from build123d import *

# Parameters (mm, degrees)
F0_R     = 2
F1_DEPTH = 3
F2_R     = 4
F3_DEPTH = 2


with BuildPart() as f1:
    # F0 (on Front) → F1 (new body)
    with BuildSketch(Plane.XZ):
        with BuildLine():
            ThreePointArc((0, 5), (1.464466, 1.464466), (5, 0))
            Line((5, 0), (70, 0))
            ThreePointArc((70, 0), (73.535534, 1.464466), (75, 5))
            Line((75, 5), (75, 20))
            ThreePointArc((75, 20), (73.535534, 23.535534), (70, 25))
            Line((70, 25), (5, 25))
            ThreePointArc((5, 25), (1.464466, 23.535534), (0, 20))
            Line((0, 20), (0, 5))
        make_face()
        with Locations((5, 5)):
            Circle(F0_R, mode=Mode.SUBTRACT)
        with Locations((70, 20)):
            Circle(F0_R, mode=Mode.SUBTRACT)
    extrude(amount=F1_DEPTH)

    # F2 (on face) → F3 (cut)
    with BuildSketch(Plane.XZ.offset(3)):
        with Locations((5, 5)):
            Circle(F2_R)
        with Locations((70, 20)):
            Circle(F2_R)
    extrude(amount=-F3_DEPTH, mode=Mode.SUBTRACT)


solid = f1.part
Check sheet for the modelled part. Datum: model origin and axes. Units: mm. A direction names the side the tool comes from. Give positions to 0.01 mm unless a question says otherwise; leave off trailing zeros. Write each loop counter-clockwise with the first axis right and the second up, starting at its lowest first coordinate (ties: lowest second). Pieces come first, ordered by that corner, then holes. Notation, with made-up numbers: (41.25, 7.25) -> (49.25, 7.25) arc R16 cw to (49.25, 13.25) -> close; hole circle Ø11 at (21.25, 5.25). An arc over 180 degrees is marked (long way). Use one line per item in the form item = value. Start each with the question number.
1. Thickness scan on line 1 along Z through (x, y) = (5, -0.4); line 2 along X through (y, z) = (-0.35, 20); line 3 along Z through (x, y) = (5, -1.95). Record the ranges inside material, lowest first. Write a range as from..to.
2. Mould release check, pull along Z, two halves, no side actions. Record for faces 3 (the flat face through (6, -1, 7)), 4 (the flat face through (37, 0, 13)), 5 (the flat face through (68, -1, 19)), 6 (the cylindrical face through (74, -1, 23)): pulls with the +Z half, pulls with the -Z half, needs draft (parallel to the pull), parting line crosses it, or undercut.
3. Section check A-A (y = -0.5). Record the cut outline in (x, z).
4. Access from +Z, -Z, +X, -X, +Y, -Y to the whole of each face (thin tool, end or side, straight path). Record for faces 1 (the flat face through (0, -1, 13)), 2 (the cylindrical face through (73.815, -2.014, 21.201)).
5. Section check B-B (z = 21). Record the cut outline in (x, y).
6. Go/stop test with flat-tipped pins: P1, Ø4, axis at x = 70, z = 21.5, coming from the -Y side; P2, Ø3, axis at x = 5, z = 5, coming from the +Y side (3 decimals). Record where each tip stops, or that it passes through.
Conclusion:
q1.line_1 = 0..3, 7..25
q1.line_2 = 0..68, 72..75
q1.line_3 = 0..1, 9..25
q2.face_3 = undercut
q2.face_4 = needs draft
q2.face_5 = undercut
q2.face_6 = pulls with the +Z half
q3.outline = (0, 5) arc R5 ccw to (5, 0) -> (70, 0) arc R5 ccw to (75, 5) -> (75, 20) arc R5 ccw to (70, 25) -> (5, 25) arc R5 ccw to (0, 20) -> close; hole circle Ø4 at (5, 5); hole circle Ø4 at (70, 20)
q4.face_1 = +Z, -Z, -X, +Y, -Y
q4.face_2 = -Y
q5.outline = (0.1, -3) -> (66.13, -3) -> (66.13, -1) -> (68.27, -1) -> (68.27, 0) -> (0.1, 0) -> close; (71.73, -1) -> (73.87, -1) -> (73.87, -3) -> (74.9, -3) -> (74.9, 0) -> (71.73, 0) -> close
q6.P1 = -1
q6.P2 = through
